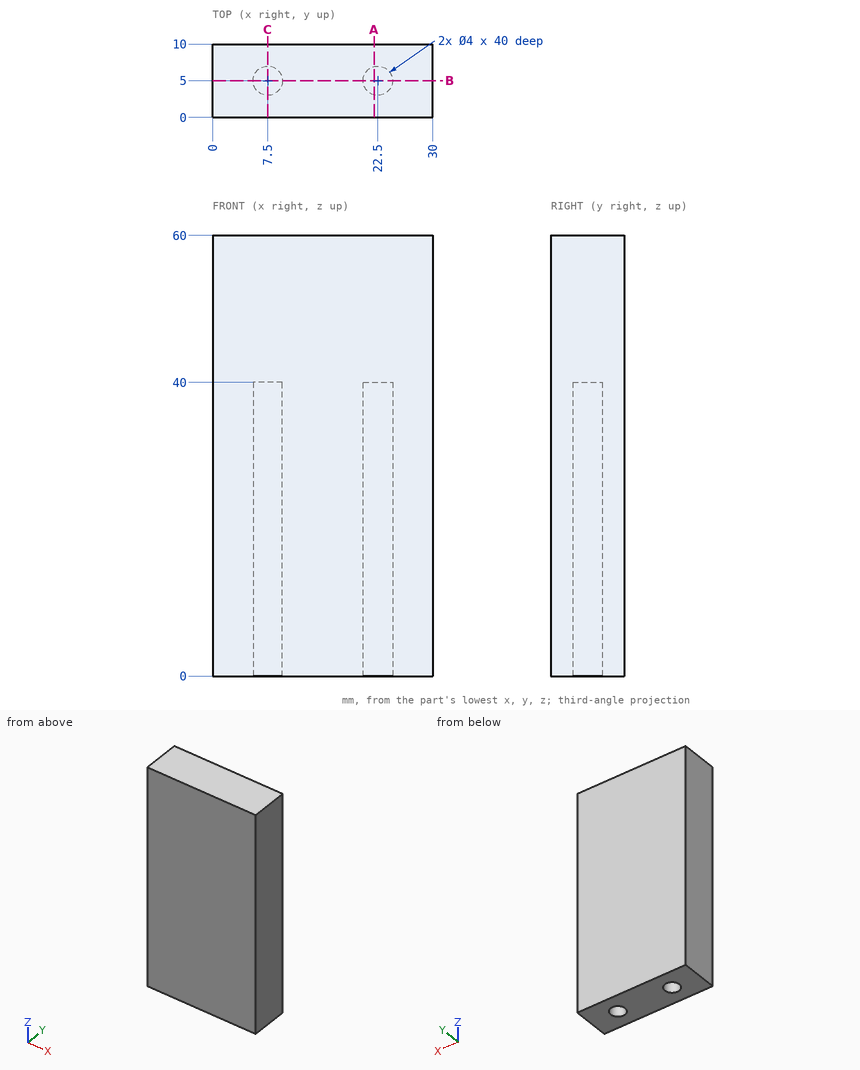
Verification items for this drawing (mm, ordinates from the low corner). Coordinates: 2 decimals unless noted, no trailing zeros. Write each loop counter-clockwise with the first axis right and the second up, starting at its lowest first coordinate (ties: lowest second). Pieces come first, ordered by that corner, then holes. Notation, with made-up numbers: M -22.75,85.25 L 28.25,85.25 A30 cw 28.25,108.25 Z; hole C 27,24 d2. An arc over 180 degrees is marked long. Answer as a JSON object with one key per item and string values.
1. Go/stop test with a flat-tipped pin: pin 1 Ø1.2 at (x, y) = (22, 5) entering from -Z. Record where the tip stops, or that it passes through.
Answers below:
{"pin 1": "stops at z = 40"}
2. Section check A-A, the plane x = 22. Enter the section's corners in (y, z).
Answers below:
{"outline": "M 0,0 L 3.06,0 L 3.06,40 L 6.94,40 L 6.94,0 L 10,0 L 10,60 L 0,60 Z"}
3. Scan lines: L1, parallel to Y at x = 7.5, z = 22; L2, parallel to X at y = 3.5, z = 18.5; L3, parallel to Y at x = 7, z = 18. Record each from-to range of solid material in increasing order.
Answers below:
{"L1": "y = 0 to 3, 7 to 10", "L2": "x = 0 to 6.18, 8.82 to 21.18, 23.82 to 30", "L3": "y = 0 to 3.06, 6.94 to 10"}
4. Section check C-C, the plane x = 7.5. Enter the section's corners in (y, z).
Answers below:
{"outline": "M 0,0 L 3,0 L 3,40 L 7,40 L 7,0 L 10,0 L 10,60 L 0,60 Z"}
5. Section check B-B, the plane y = 5. Enter the section's corners in (x, z), plus the area to 3 significant figures.
Answers below:
{"outline": "M 0,0 L 5.5,0 L 5.5,40 L 9.5,40 L 9.5,0 L 20.5,0 L 20.5,40 L 24.5,40 L 24.5,0 L 30,0 L 30,60 L 0,60 Z", "area": "1,480 mm²"}
